```python
from build123d import *

# Parameters (mm, degrees)
BOSS_EXTRUDE1_DEPTH = 10
SKETCH2_W           = 20
SKETCH2_H           = 5
BOSS_EXTRUDE2_DEPTH = 15
FILLET3_R           = 5
FILLET4_R           = 5
BOSS_EXTRUDE4_DEPTH = 5
SKETCH4_R           = 5
CUT_EXTRUDE1_DEPTH  = 5


with BuildPart() as part:
    # Sketch1 → Boss-Extrude1 (new body)
    with BuildSketch(Plane.XY):
        with BuildLine():
            Line((-10, -15), (-10, -10))
            ThreePointArc((-10, -10), (0, 0), (10, -10))
            Line((10, -10), (10, -15))
            Line((10, -15), (25, -15))
            ThreePointArc((25, -15), (32.071067812, -12.071067812), (35, -5))
            Line((35, -5), (35, 5))
            ThreePointArc((35, 5), (32.071067812, 12.071067812), (25, 15))
            Line((25, 15), (-25, 15))
            ThreePointArc((-25, 15), (-32.071067812, 12.071067812), (-35, 5))
            Line((-35, 5), (-35, -5))
            ThreePointArc((-35, -5), (-32.071067812, -12.071067812), (-25, -15))
            Line((-25, -15), (-10, -15))
        make_face()
        with BuildLine():
            Line((30, 7.354167283), (30, -2.645832717))
            ThreePointArc((30, -2.645832717), (25, -7.645832717), (20, -2.645832717))
            Line((20, -2.645832717), (20, 7.354167283))
            ThreePointArc((20, 7.354167283), (25, 12.354167283), (30, 7.354167283))
        make_face(mode=Mode.SUBTRACT)
        with BuildLine():
            Line((-20, 7.354167283), (-20, -2.645832717))
            ThreePointArc((-20, -2.645832717), (-25, -7.645832717), (-30, -2.645832717))
            Line((-30, -2.645832717), (-30, 7.354167283))
            ThreePointArc((-30, 7.354167283), (-25, 12.354167283), (-20, 7.354167283))
        make_face(mode=Mode.SUBTRACT)
    extrude(amount=BOSS_EXTRUDE1_DEPTH)

    # Sketch2 → Boss-Extrude2 (add)
    with BuildSketch(Plane.XY.offset(10)):
        with Locations((0, 12.5)):
            Rectangle(SKETCH2_W, SKETCH2_H)
    extrude(amount=BOSS_EXTRUDE2_DEPTH)

    # Fillet3
    fillet3_edges = [part.edges().sort_by_distance(p)[0] for p in [
        (-10, 12.5, 10),
    ]]
    fillet(fillet3_edges, radius=FILLET3_R)

    # Fillet4
    fillet4_edges = [part.edges().sort_by_distance(p)[0] for p in [
        (10, 12.5, 10),
    ]]
    fillet(fillet4_edges, radius=FILLET4_R)

    # Sketch3 → Boss-Extrude4 (add)
    with BuildSketch(Plane(origin=(0, 15, 0), x_dir=(1, 0, 0), z_dir=(0, 1, 0))):
        with BuildLine():
            Line((-10, -25), (10, -25))
            ThreePointArc((10, -25), (0, -35), (-10, -25))
        make_face()
    extrude(amount=-BOSS_EXTRUDE4_DEPTH)

    # Sketch4 → Cut-Extrude1 (cut)
    with BuildSketch(Plane(origin=(0, 15, 0), x_dir=(1, 0, 0), z_dir=(0, 1, 0))):
        with Locations(Location((0, -25, 0), (0, 0, 270))):
            Circle(SKETCH4_R)
    extrude(amount=-CUT_EXTRUDE1_DEPTH, mode=Mode.SUBTRACT)


solid = part.part
```
Verification items for the finished model (mm, model axes). A direction names the side the tool comes from. Give positions to 0.01 mm unless a question says otherwise; leave off trailing zeros. Order: outer loops, then holes, each group sorted by start corner. A loop starts at its lowest first (then second) coordinate and runs counter-clockwise, first axis right, second up. Notation, with made-up numbers: (15.5, 38.25) - (25.5, 38.25) arc R11 cw to (25.5, 52.25) - close; hole circle Ø11 at (-10, -2.75). An arc over 180 degrees is marked (long way). Answer as CSV lines item,"result". Start each with the question number.
Item 1: Section check D-D, the plane y = -4. Record the boundary of the cut face in (x, z).
Item 2: Section check B-B, the plane z = 7. Record the boundary of the cut face in (x, y).
Item 3: Gauge pin test, flat ends, axial feed: pin 1 (1 mm diameter, centred on x = -21, y = 0, fed in from +Z); pin 2 (2.5 mm diameter, centred on y = -13.5, z = 3.5, fed in from -X); pin 3 (5 mm diameter, centred on x = 7.5, z = 30.5, fed in from -Y); pin 4 (5.5 mm diameter, centred on y = 13.5, z = 22, fed in from +X). Record the tip position at first contact, or that the pin passes through.
Item 4: Section check C-C, the plane y = -8.5. Record the boundary of the cut face in (x, z), plus the area to 3 significant figures.
Item 5: Material ranges on L1, parallel to X at y = 12.55, z = 25; L2, parallel to Y at x = 5.5, z = 29.5; L3, parallel to Z at x = 25, y = -9, recorded low to high.
Item 6: Mould release check, pull along Y, two halves, no side actions. Record for faces 1 (the face through (-18, -15, 5)), 2 (the face through (35, 0, 5)), 3 (the face through (25.11, -7.645, 4.93)): released by +Y, released by -Y, zero draft, split by the parting line, or undercut.
Item 7: Access from +Z, -Z, +X, -X, +Y, -Y to the whole of each face (thin tool, end or side, straight path). Record for faces 4 (the face through (-30, 2, 5)), 5 (the face through (-10, 12, 20)), 6 (the face through (-10, -13, 5)).
Item 8: Section check A-A, the plane x = 0. Record the boundary of the cut face in (y, z).
Filled in:
1,outline,"(-35, 0) - (-29.81, 0) - (-29.81, 10) - (-35, 10) - close; (-20.19, 0) - (-8, 0) - (-8, 10) - (-20.19, 10) - close; (8, 0) - (20.19, 0) - (20.19, 10) - (8, 10) - close; (29.81, 0) - (35, 0) - (35, 10) - (29.81, 10) - close"
2,outline,"(-35, -5) arc R10 ccw to (-25, -15) - (-10, -15) - (-10, -10) arc R10 cw to (10, -10) - (10, -15) - (25, -15) arc R10 ccw to (35, -5) - (35, 5) arc R10 ccw to (25, 15) - (-25, 15) arc R10 ccw to (-35, 5) - close; hole (-30, -2.65) arc R5 ccw to (-20, -2.65) - (-20, 7.35) arc R5 ccw to (-30, 7.35) - close; hole (20, -2.65) arc R5 ccw to (30, -2.65) - (30, 7.35) arc R5 ccw to (20, 7.35) - close"
3,pin 1,"through"
3,pin 2,"x = -31.89"
3,pin 3,"y = 10"
3,pin 4,"x = 10"
4,outline,"(-34.37, 0) - (-9.89, 0) - (-9.89, 10) - (-34.37, 10) - close; (9.89, 0) - (34.37, 0) - (34.37, 10) - (9.89, 10) - close"
4,area,"490 mm^2"
5,L1,"-10 to -5, 5 to 10"
5,L2,"10 to 15"
5,L3,"0 to 10"
6,face 1,"released by -Y"
6,face 2,"zero draft"
6,face 3,"undercut"
7,face 4,"+Z, -Z"
7,face 5,"+Z, -X, +Y, -Y"
7,face 6,"+Z, -Z, -Y"
8,outline,"(0, 0) - (15, 0) - (15, 20) - (10, 20) - (10, 10) - (0, 10) - close; (10, 30) - (15, 30) - (15, 35) - (10, 35) - close"
